from build123d import *

# Parameters (mm, degrees)
F0_W     = 2.667
F0_H     = 8.255
F1_DEPTH = 2.54
F2_DEPTH = 2.54
F3_DEPTH = 11.303


with BuildPart() as f1:
    # F0 (on Front) → F1 (new body)
    with BuildSketch(Plane.XZ):
        with BuildLine():
            Line((40.015628993, 17.0561), (22.057944681, 17.0561))
            ThreePointArc((22.057944681, 17.0561), (26.9348097233, 9.1403911713), (28.636428993, 0))
            ThreePointArc((28.636428993, 0), (26.9348097233, -9.1403911713), (22.057944681, -17.0561))
            Line((22.057944681, -17.0561), (40.015628993, -17.0561))
            Line((40.015628993, -17.0561), (40.015628993, 0))
            Line((40.015628993, 0), (40.015628993, 17.0561))
        make_face()
        with Locations((-48.820871007, 14.2875)):
            Rectangle(F0_W, F0_H)
        with BuildLine():
            Line((-3.672371007, 21.082), (-12.511571007, 21.082))
            Line((-12.511571007, 21.082), (-12.511571007, 6.2905908912))
            ThreePointArc((-12.511571007, 6.2905908912), (-10.276371007, 0), (-12.511571007, -6.2905908912))
            Line((-12.511571007, -6.2905908912), (-12.511571007, -21.082))
            Line((-12.511571007, -21.082), (-3.672371007, -21.082))
            Line((-3.672371007, -21.082), (-2.529371007, -17.0561))
            Line((-2.529371007, -17.0561), (22.057944681, -17.0561))
            ThreePointArc((22.057944681, -17.0561), (26.9348097233, -9.1403911713), (28.636428993, 0))
            ThreePointArc((28.636428993, 0), (26.9348097233, 9.1403911713), (22.057944681, 17.0561))
            Line((22.057944681, 17.0561), (-2.529371007, 17.0561))
            Line((-2.529371007, 17.0561), (-3.672371007, 21.082))
        make_face()
        with BuildLine():
            ThreePointArc((-12.511571007, -6.2905908912), (-10.276371007, 0), (-12.511571007, 6.2905908912))
            Line((-12.511571007, 6.2905908912), (-12.511571007, 0))
            Line((-12.511571007, 0), (-12.511571007, -6.2905908912))
        make_face()
        with BuildLine():
            Line((-12.511571007, 21.082), (-47.487371007, 21.082))
            Line((-47.487371007, 21.082), (-47.487371007, 18.415))
            Line((-47.487371007, 18.415), (-47.487371007, 10.16))
            Line((-47.487371007, 10.16), (-47.487371007, 0))
            Line((-47.487371007, 0), (-47.487371007, -10.16))
            Line((-47.487371007, -10.16), (-47.487371007, -18.415))
            Line((-47.487371007, -18.415), (-47.487371007, -21.082))
            Line((-47.487371007, -21.082), (-12.511571007, -21.082))
            Line((-12.511571007, -21.082), (-12.511571007, -6.2905908912))
            ThreePointArc((-12.511571007, -6.2905908912), (-15.9635302708, -9.0029155316), (-20.245871007, -9.9695))
            Line((-20.245871007, -9.9695), (-33.707871007, -9.9695))
            ThreePointArc((-33.707871007, -9.9695), (-43.677371007, 0), (-33.707871007, 9.9695))
            Line((-33.707871007, 9.9695), (-20.245871007, 9.9695))
            ThreePointArc((-20.245871007, 9.9695), (-15.9635302708, 9.0029155316), (-12.511571007, 6.2905908912))
            Line((-12.511571007, 6.2905908912), (-12.511571007, 21.082))
        make_face()
        with Locations((-48.820871007, -14.2875)):
            Rectangle(F0_W, F0_H)
    extrude(amount=-F1_DEPTH)

    # F0 (on Front) → F2 (join)
    with BuildSketch(Plane.XZ):
        with BuildLine():
            Line((-3.672371007, 21.082), (-12.511571007, 21.082))
            Line((-12.511571007, 21.082), (-12.511571007, 6.2905908912))
            ThreePointArc((-12.511571007, 6.2905908912), (-10.276371007, 0), (-12.511571007, -6.2905908912))
            Line((-12.511571007, -6.2905908912), (-12.511571007, -21.082))
            Line((-12.511571007, -21.082), (-3.672371007, -21.082))
            Line((-3.672371007, -21.082), (-2.529371007, -17.0561))
            Line((-2.529371007, -17.0561), (22.057944681, -17.0561))
            ThreePointArc((22.057944681, -17.0561), (26.9348097233, -9.1403911713), (28.636428993, 0))
            ThreePointArc((28.636428993, 0), (26.9348097233, 9.1403911713), (22.057944681, 17.0561))
            Line((22.057944681, 17.0561), (-2.529371007, 17.0561))
            Line((-2.529371007, 17.0561), (-3.672371007, 21.082))
        make_face()
        with BuildLine():
            ThreePointArc((-12.511571007, -6.2905908912), (-10.276371007, 0), (-12.511571007, 6.2905908912))
            Line((-12.511571007, 6.2905908912), (-12.511571007, 0))
            Line((-12.511571007, 0), (-12.511571007, -6.2905908912))
        make_face()
        with BuildLine():
            Line((17.4036191167, 21.082), (-3.672371007, 21.082))
            Line((-3.672371007, 21.082), (-2.529371007, 17.0561))
            Line((-2.529371007, 17.0561), (22.057944681, 17.0561))
            ThreePointArc((22.057944681, 17.0561), (19.8531568744, 19.2105271796), (17.4036191167, 21.082))
        make_face()
        with BuildLine():
            Line((-2.529371007, -17.0561), (-3.672371007, -21.082))
            Line((-3.672371007, -21.082), (17.4036191167, -21.082))
            ThreePointArc((17.4036191167, -21.082), (19.8531568744, -19.2105271796), (22.057944681, -17.0561))
            Line((22.057944681, -17.0561), (-2.529371007, -17.0561))
        make_face()
    extrude(amount=F2_DEPTH)

    # F0 (on Front) → F3 (join)
    with BuildSketch(Plane.XZ):
        with Locations((-48.820871007, 14.2875)):
            Rectangle(F0_W, F0_H)
        with Locations((-48.820871007, -14.2875)):
            Rectangle(F0_W, F0_H)
    extrude(amount=-F3_DEPTH)


solid = f1.part
Read the model definition and answer for the solid it produces. Units are mm, in the model's axes. A direction names the side the tool comes from. Give positions to 0.01 mm unless a question says otherwise; leave off trailing zeros. Write each loop counter-clockwise with the first axis right and the second up, starting at its lowest first coordinate (ties: lowest second). Pieces come first, ordered by that corner, then holes. Notation, with made-up numbers: M 1.5,-19.75 L 50.5,-19.75 A37 cw 50.5,16.25 Z; hole C -27.75,-6 d6. An arc over 180 degrees is marked long. One line per item, written item: value. Start each with the question number.
(1) Flat-ended cylindrical pins translate along their axes: pin 1 Ø0.8 at (y, z) = (1.5, -20) entering from -X; pin 2 Ø1.3 at (x, y) = (26, 1.5) entering from +Z; pin 3 Ø6.5 at (y, z) = (7.5, 15.5) entering from +X. Find the tip coordinate at first contact, or state that the pin passes through.
(2) Find section A-A (y = 5.75). Determine the outline of the cut face in (x, z) (3 decimals), plus the area to 3 significant figures.
(3) Find the intervals of material crossed by line 1 (Y direction, x = 15.5, z = -16); line 2 (X direction, y = 4.25, z = -13.5); line 3 (X direction, y = 0.25, z = -6), in increasing order.
(4) Find section D-D (y = 1). Determine the outline of the cut face in (x, z) (1 decimal), plus the area to 3 significant figures.
(5) A tool of negligible diameter and unlimited length cuts with its end or side. For faces 5 (the cylindrical face through (-43.675, 1.252, -0.219)), 6 (the flat face through (-12.512, -1, 0)), 7 (the flat face through (-49, 6, -10.16)), 8 (the flat face through (-47.487, 7, -14)), from which of +Z, -Z, +X, -X, +Y, -Y can it reach the whole face along a straight path? Write none if from no direction.
(6) Determine the mould class of faces 1 (the cylindrical face through (-15.908, 1.252, -8.976)), 2 (the flat face through (-27, 1, 9.97)), 3 (the flat face through (-50.154, 6, 14)), 4 (the flat face through (-49, 11.303, -14)) for opening direction X: pulls with the +X half, pulls with the -X half, needs draft (parallel to the pull), parting line crosses it, or undercut.
(7) Find section B-B (z = 9). Determine the outline of the cut face in (x, y).
(8) Find section C-C (x = -39). Determine the outline of the cut face in (y, z).
Results below:
1. pin 1: stops at x = -47.49
1. pin 2: stops at z = 17.06
1. pin 3: stops at x = -47.49
2. outline: M -50.154,-18.415 L -47.487,-18.415 L -47.487,-10.16 L -50.154,-10.16 Z; M -50.154,10.16 L -47.487,10.16 L -47.487,18.415 L -50.154,18.415 Z
2. area: 44.0 mm^2
3. line 1: y = -2.54 to 2.54
3. line 2: x = -50.15 to -47.49
3. line 3: x = -47.49 to -41.67, -12.51 to 40.02
4. outline: M -50.2,-18.4 L -47.5,-18.4 L -47.5,-21.1 L -3.7,-21.1 L -2.5,-17.1 L 40,-17.1 L 40,17.1 L -2.5,17.1 L -3.7,21.1 L -47.5,21.1 L -47.5,18.4 L -50.2,18.4 L -50.2,10.2 L -47.5,10.2 L -47.5,-10.2 L -50.2,-10.2 Z; hole M -33.7,-10 L -20.2,-10 A10 ccw -12.5,-6.3 L -12.5,6.3 A10 ccw -20.2,10 L -33.7,10 A10 ccw Z
4. area: 2,820 mm^2
5. face 5: +Y, -Y
5. face 6: -Y
5. face 7: -X, +Y, -Y
5. face 8: +Z, -Z, +X, +Y
6. face 1: undercut
6. face 2: undercut
6. face 3: pulls with the -X half
6. face 4: needs draft
7. outline: M -47.49,0 L -38,0 L -38,2.54 L -47.49,2.54 Z; M -15.96,0 L -12.51,0 L -12.51,-2.54 L 26.99,-2.54 L 26.99,0 L 40.02,0 L 40.02,2.54 L -15.96,2.54 Z
8. outline: M 0,-21.08 L 2.54,-21.08 L 2.54,-8.45 L 0,-8.45 Z; M 0,8.45 L 2.54,8.45 L 2.54,21.08 L 0,21.08 Z
